For this review, take the finished solid that the model builds, in its own axes (mm). A direction names the side the tool comes from. Round coordinates to 2 decimals unless told otherwise and drop trailing zeros. Loops run counter-clockwise (first coordinate to the right, second up) from the corner with the lowest first, then second, coordinate; pieces in that order, holes last.
1. Draft analysis for pull direction Y (two halves, no side actions). For faces 1 (the flat face through (-0.99, -18.68, 19.79)), 2 (the flat face through (130.1, -23, 27)), 3 (the flat face through (120.2, -14, 9)), state which applies: released by +Y, released by -Y, zero draft, split by the parting line, or undercut.
2. Consider section D-D on z = 0. State the section outline as (x, y) points, then the cut area to 3 significant figures.
3. Consider section C-C on x = 57.5. State the section outline as (y, z) points, then the cut area to 3 significant figures.
4. Tool access review of faces 4 (the flat face through (122.2, -14, 9)), 5 (the flat face through (-0.99, -11.74, -1.33)), 6 (the flat face through (-2, -14, 9)), 7 (the flat face through (0, -14, 9)): name each direction out of +Z, -Z, +X, -X, +Y, -Y from which nothing blocks a thin tool from reaching the whole face with its end or side.
5. Consider section B-B on y = -9.5. State the section outline as (x, z) points, then the cut area to 3 significant figures.
6. To check wall thickness, follow line 1 along X through (y, z) = (-8, 4.5); line 2 along Z through (x, y) = (36, -23.5); line 3 along Z through (x, y) = (106, -20). State the ranges of each line that lie inside material, in increasing order.
7. Clearance check with flat-ended pins moving along their axes: pin 1 Ø5 at (x, y) = (20.5, -12) entering from -Z; pin 2 Ø4 at (x, y) = (12.5, -17.5) entering from +Z; pin 3 Ø10 at (x, z) = (92.5, 21) entering from +Y; pin 4 Ø3 at (x, z) = (76, -1.5) entering from -Y. State where each tip first meets the part, or that it passes through.
8. Consider section A-A on z = 18. State the section outline as (x, y) points.
from build123d import *
from build123d.topology import SkipClean

# Parameters (mm, degrees)
CROQUIS1_R                = 5
SALIENTE_EXTRUIR6_DEPTH   = 120.2
SALIENTE_EXTRUIR6_2_DEPTH = 120.2
CROQUIS1_R_2              = 2
SALIENTE_EXTRUIR6_3_DEPTH = 120.2
SALIENTE_EXTRUIR8_DEPTH   = 2
SALIENTE_EXTRUIR9_DEPTH   = 2
SALIENTE_EXTRUIR10_DEPTH  = 7.9
CROQUIS14_R               = 5
CROQUIS14_R_2             = 2
SALIENTE_EXTRUIR11_DEPTH  = 7.9


with BuildPart() as part:
    # Croquis1 → Saliente-Extruir6 (new body)
    with BuildSketch(Plane(origin=(0, 0, 0), x_dir=(0, 0, -1), z_dir=(1, 0, 0))):
        Circle(CROQUIS1_R)
    extrude(amount=SALIENTE_EXTRUIR6_DEPTH)



with BuildPart() as body_2:
    # Croquis1 → Saliente-Extruir6 2 (new body)
    with BuildSketch(Plane(origin=(0, 0, 0), x_dir=(0, 0, -1), z_dir=(1, 0, 0))):
        with Locations((-6.915082, -20.579255)):
            Circle(CROQUIS1_R)
    extrude(amount=SALIENTE_EXTRUIR6_2_DEPTH)


with BuildPart() as body_3:
    # Croquis1 → Saliente-Extruir6 3 (new body)
    with BuildSketch(Plane(origin=(0, 0, 0), x_dir=(0, 0, -1), z_dir=(1, 0, 0))):
        with Locations((-27.035927, -22.579255)):
            Circle(CROQUIS1_R_2)
    extrude(amount=SALIENTE_EXTRUIR6_3_DEPTH)


with BuildPart() as part_1:
    with SkipClean():  # the faces are left unmerged after this step: merging them gives an invalid solid
        add(part.part)

        add(body_2.part)  # Saliente-Extruir8 merges body 2

        add(body_3.part)  # Saliente-Extruir8 merges body 3
        # Croquis10 → Saliente-Extruir8 (add)
        with BuildSketch(Plane.ZY):
            with BuildLine():
                Line((-4.73958, -1.592603), (2.175502, -22.171858))
                ThreePointArc((2.175502, -22.171858), (4.098509, -24.710467), (7.164198, -25.573045))
                Line((7.164198, -25.573045), (27.135573, -24.576771))
                ThreePointArc((27.135573, -24.576771), (29.026119, -22.777079), (27.526842, -20.64044))
                Line((27.526842, -20.64044), (11.843492, -16.669357))
                ThreePointArc((11.843492, -16.669357), (10.975071, -16.197582), (10.438575, -15.367583))
                Line((10.438575, -15.367583), (4.73958, 1.592603))
                ThreePointArc((4.73958, 1.592603), (-1.592603, 4.73958), (-4.73958, -1.592603))
            make_face()
        extrude(amount=SALIENTE_EXTRUIR8_DEPTH)

    # Croquis11 → Saliente-Extruir9 (add)
    with BuildSketch(Plane(origin=(120.2, 0, 0), x_dir=(0, 0, -1), z_dir=(1, 0, 0))):
        with BuildLine():
            Line((4.73958, -1.592603), (-2.175502, -22.171858))
            ThreePointArc((-2.175502, -22.171858), (-4.098509, -24.710467), (-7.164198, -25.573045))
            Line((-7.164198, -25.573045), (-27.135573, -24.576771))
            ThreePointArc((-27.135573, -24.576771), (-29.026119, -22.777079), (-27.526842, -20.64044))
            Line((-27.526842, -20.64044), (-11.843492, -16.669357))
            ThreePointArc((-11.843492, -16.669357), (-10.975071, -16.197582), (-10.438575, -15.367583))
            Line((-10.438575, -15.367583), (-4.73958, 1.592603))
            ThreePointArc((-4.73958, 1.592603), (1.592603, 4.73958), (4.73958, -1.592603))
        make_face()
    extrude(amount=SALIENTE_EXTRUIR9_DEPTH)

    # Croquis13 → Saliente-Extruir10 (add)
    with BuildSketch(Plane(origin=(122.2, 0, 0), x_dir=(0, 0, -1), z_dir=(1, 0, 0))):
        with BuildLine():
            ThreePointArc((-7.164198, -25.573045), (-4.098509, -24.710467), (-2.175502, -22.171858))
            ThreePointArc((-2.175502, -22.171858), (-1.980616, -21.386132), (-1.915082, -20.579255))
            ThreePointArc((-1.915082, -20.579255), (-10.361415, -16.956716), (-7.164198, -25.573045))
        make_face()
        with BuildLine():
            ThreePointArc((5, 0), (0.806877, 4.934465), (-4.73958, 1.592603))
            ThreePointArc((-4.73958, 1.592603), (-1.592603, -4.73958), (4.73958, -1.592603))
            ThreePointArc((4.73958, -1.592603), (4.934465, -0.806877), (5, 0))
        make_face()
        with BuildLine():
            ThreePointArc((-25.035927, -22.579255), (-25.807479, -21.000992), (-27.526842, -20.64044))
            ThreePointArc((-27.526842, -20.64044), (-29.026119, -22.777079), (-27.135573, -24.576771))
            ThreePointArc((-27.135573, -24.576771), (-25.657394, -24.028271), (-25.035927, -22.579255))
        make_face()
    extrude(amount=SALIENTE_EXTRUIR10_DEPTH)

    # Croquis14 → Saliente-Extruir11 (add)
    with BuildSketch(Plane.ZY.offset(2)):
        Circle(CROQUIS14_R)
        with Locations(Location((27.035927, -22.579255, 0), (0, 0, 180))):
            Circle(CROQUIS14_R_2)
        with Locations(Location((6.915082, -20.579255, 0), (0, 0, 180))):
            Circle(CROQUIS14_R)
    extrude(amount=SALIENTE_EXTRUIR11_DEPTH)


solid = part_1.part
Resolved:
1. face 1: released by +Y
1. face 2: zero draft
1. face 3: undercut
2. outline: (-9.9, -5) - (-2, -5) - (-2, -15.7) - (0, -15.7) - (0, -5) - (120.2, -5) - (120.2, -15.7) - (122.2, -15.7) - (122.2, -5) - (130.1, -5) - (130.1, 5) - (-9.9, 5) - close
2. area: 1,440 mm2
3. outline: circle Ø10 at (-20.58, 6.92); circle Ø4 at (-22.58, 27.04); circle Ø10 at (0, 0)
3. area: 170 mm2
4. face 4: +X
4. face 5: -Z, +X, -X, -Y
4. face 6: -X
4. face 7: none
5. outline: (-2, -2.08) - (0, -2.08) - (0, 8.47) - (-2, 8.47) - close; (120.2, -2.08) - (122.2, -2.08) - (122.2, 8.47) - (120.2, 8.47) - close
5. area: 42.2 mm2
6. line 1: x = -2 to 0, 120.2 to 122.2
6. line 2: z = 2.86 to 10.97, 25.26 to 28.81
6. line 3: z = 1.95 to 11.88
7. pin 1: passes through
7. pin 2: stops at z = 11.8
7. pin 3: stops at y = -20.87
7. pin 4: stops at y = -5
8. outline: (-2, -25.03) - (0, -25.03) - (0, -18.23) - (-2, -18.23) - close; (120.2, -25.03) - (122.2, -25.03) - (122.2, -18.23) - (120.2, -18.23) - close
